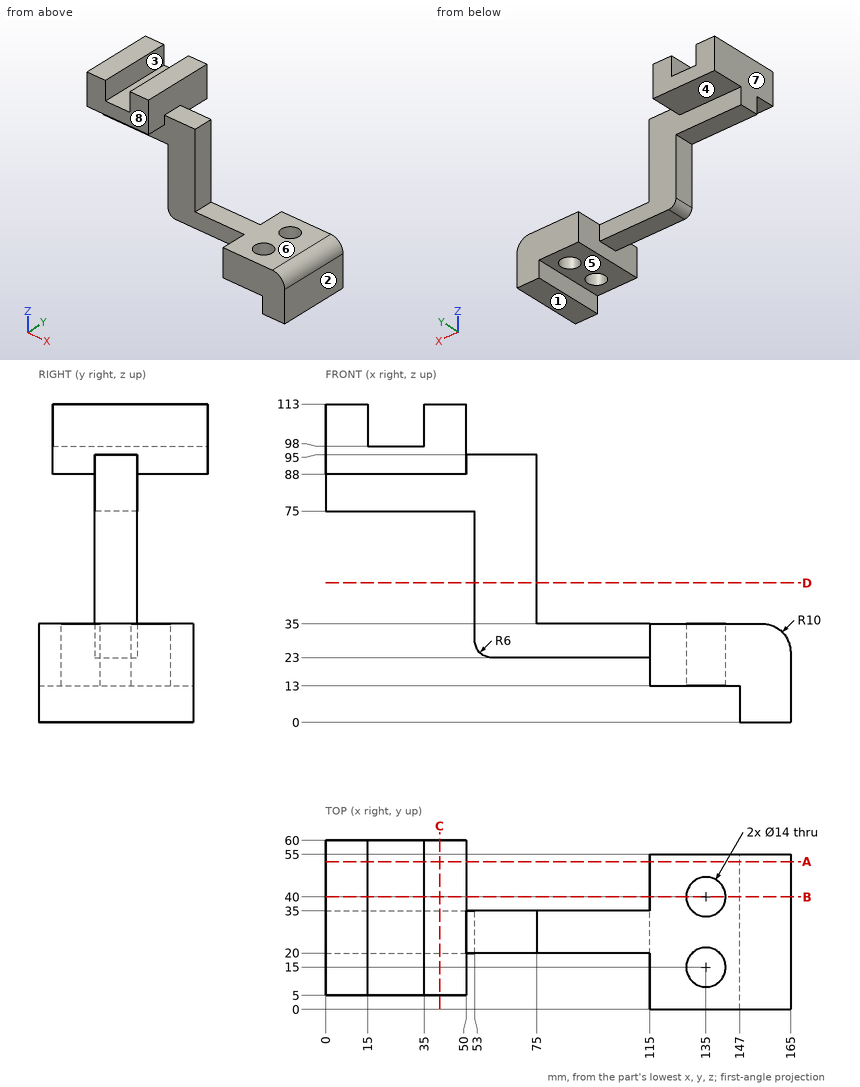
The drawing under review shows one solid part. Ordinate dimensions are in mm from its lowest x, y, z. A direction names the side the tool comes from. Give positions to 0.01 mm unless a question says otherwise; leave off trailing zeros. Order: outer loops, then holes, each group sorted by start corner. A loop starts at its lowest first (then second) coordinate and runs counter-clockwise, first axis right, second up. Notation, with made-up numbers: M 13,15 L 71,15 A21 ccw 71,42 Z; hole C 37,-17.75 d11. An arc over 180 degrees is marked long. Answer in a Markdown table with one row per item. Add a question column.
1. Machinability: for the marked faces 4, 5, 6, 7 and 8, which of the approach directions +Z, -Z, +X, -X, +Y, -Y give a long, thin tool a straight path to every point of the face, cutting with its end or side? Answer none if there is none.
2. Add section D-D on z = 49.5. State the section outline as (x, y) points.
3. Mouldability with a two-part tool opening along X and no side actions: class the marked faces 1, 2 and 3 as released by +X, released by -X, zero draft, split by the parting line, or undercut.
4. To check wall thickness, follow line 1 along X through (y, z) = (40, 22); line 2 along X through (y, z) = (15.5, 100.5); line 3 along Y through (x, z) = (118, 14). State the ranges of each line that lie inside material, in increasing order.
5. For pin 1 Ø7.5 at (y, z) = (31, 109) entering from -X; pin 2 Ø12 at (x, y) = (26, 9.5) entering from -Z; pin 3 Ø12 at (x, y) = (146.5, 11) entering from +Z; pin 4 Ø7.5 at (x, y) = (65.5, 30.5) entering from +Z, all flat-tipped, find the tip position at first contact; note any pin that passes through.
6. Add section A-A on y = 52.5. State the section outline as (x, z) points, plus the area to 3 significant figures.
7. Add section B-B on y = 40. State the section outline as (x, z) points, plus the area to 3 significant figures.
8. Add section C-C on x = 40.5. State the section outline as (y, z) points.
The answers:
| question | item | result |
|---|---|---|
| 1 | face 4 | -Z, +X, -X, +Y |
| 1 | face 5 | -Z, -X, +Y, -Y |
| 1 | face 6 | +Z, +X, +Y, -Y |
| 1 | face 7 | +Z, -Z, -X, +Y, -Y |
| 1 | face 8 | +Z, -Z, +X, -X, -Y |
| 2 | outline | M 53,20 L 75,20 L 75,35 L 53,35 Z |
| 3 | face 1 | zero draft |
| 3 | face 2 | released by +X |
| 3 | face 3 | undercut |
| 4 | line 1 | 115 to 128, 142 to 165 |
| 4 | line 2 | 0 to 15, 35 to 50 |
| 4 | line 3 | 0 to 55 |
| 5 | pin 1 | x = 0 |
| 5 | pin 2 | z = 88 |
| 5 | pin 3 | z = 35 |
| 5 | pin 4 | z = 95 |
| 6 | outline | M 0,88 L 50,88 L 50,113 L 35,113 L 35,98 L 15,98 L 15,113 L 0,113 Z; M 115,13 L 147,13 L 147,0 L 165,0 L 165,25 A10 ccw 155,35 L 115,35 Z |
| 6 | area | 2,260 mm2 |
| 7 | outline | M 0,88 L 50,88 L 50,113 L 35,113 L 35,98 L 15,98 L 15,113 L 0,113 Z; M 115,13 L 128,13 L 128,35 L 115,35 Z; M 142,13 L 147,13 L 147,0 L 165,0 L 165,25 A10 ccw 155,35 L 142,35 Z |
| 7 | area | 1,950 mm2 |
| 8 | outline | M 5,88 L 20,88 L 20,75 L 35,75 L 35,88 L 60,88 L 60,113 L 5,113 Z |
